from build123d import *

# Parameters (mm, degrees)
F0_R     = 20
F1_DEPTH = 1.5
F2_R     = 17.5
F3_DEPTH = 10
F4_R     = 20
F5_DEPTH = 1.5
F6_R     = 12.5
F7_DEPTH = 5
F8_R     = 4
F9_DEPTH = 20


with BuildPart() as f1:
    # F0 (on Front) → F1 (new body)
    with BuildSketch(Plane.XZ):
        Circle(F0_R)
    extrude(amount=F1_DEPTH)

    # F2 (on face) → F3 (join)
    with BuildSketch(Plane.XZ.offset(1.5)):
        Circle(F2_R)
    extrude(amount=F3_DEPTH)

    # F4 (on face) → F5 (join)
    with BuildSketch(Plane.XZ.offset(11.5)):
        Circle(F4_R)
    extrude(amount=F5_DEPTH)

    # F6 (on face) → F7 (join)
    with BuildSketch(Plane.XZ.offset(13)):
        Circle(F6_R)
    extrude(amount=F7_DEPTH)

    # F8 (on face) → F9 (cut)
    with BuildSketch(Plane.XZ.offset(18)):
        Circle(F8_R)
    extrude(amount=-F9_DEPTH, mode=Mode.SUBTRACT)


solid = f1.part
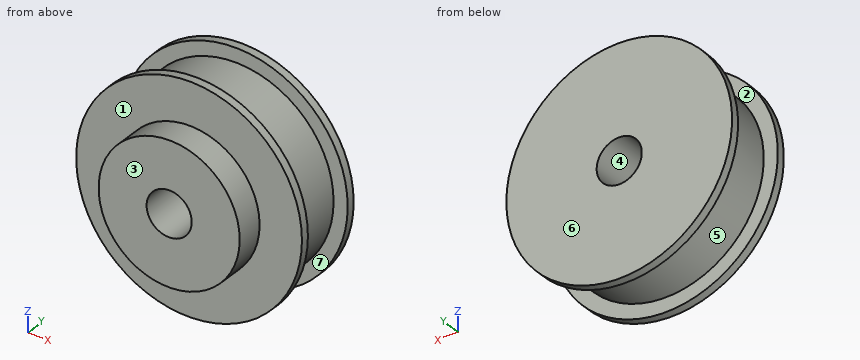
Model file for the job. Use its own axes, mm. Face numbers are marked on the shaded views. A direction names the side the tool comes from. Give positions to 0.01 mm unless a question says otherwise; leave off trailing zeros. Write each loop counter-clockwise with the first axis right and the second up, starting at its lowest first coordinate (ties: lowest second). Pieces come first, ordered by that corner, then holes. Notation, with made-up numbers: (35.5, 2.25) -> (41.5, 2.25) arc R27 ccw to (41.5, 33.25) -> close; hole circle Ø2 at (88.25, 4). An arc over 180 degrees is marked (long way). Write item = value, one per line.
(1) Slice it at C-C, the plane y = -6.5. Give the cut face in (x, z), then the cut area to 3 significant figures.
Determined:
outline = circle Ø35 at (0, 0); hole circle Ø8 at (0, 0)
area = 912 mm2
(2) Slice it at B-B, the plane x = 0. Give the cut face in (y, z).
Determined:
outline = (-18, -12.5) -> (-13, -12.5) -> (-13, -20) -> (-11.5, -20) -> (-11.5, -17.5) -> (-1.5, -17.5) -> (-1.5, -20) -> (0, -20) -> (0, -4) -> (-18, -4) -> close; (-18, 4) -> (0, 4) -> (0, 20) -> (-1.5, 20) -> (-1.5, 17.5) -> (-11.5, 17.5) -> (-11.5, 20) -> (-13, 20) -> (-13, 12.5) -> (-18, 12.5) -> close
(3) Flat gauge pins, fed straight in: P1, Ø4, axis at y = -2, z = -9, coming from the -X side; P2, Ø2, axis at x = -9.5, y = -3.5, coming from the +Z side; P3, Ø1.5, axis at x = 13, z = 5.5, coming from the -Y side; P4, Ø6.5, axis at x = 0, z = 0, coming from the -Y side. Where does each tip first touch, or does it go through?
Determined:
P1 = -18.71
P2 = 15.3
P3 = -13
P4 = through
(4) Probe line 1 along Y through (x, z) = (-6.5, 18); line 2 along Z through (x, y) = (0, -6); line 3 along Y through (x, z) = (-9, -9.5). List the from-to ranges inside material, lowest first.
Determined:
line_1 = -13 to -11.5, -1.5 to 0
line_2 = -17.5 to -4, 4 to 17.5
line_3 = -13 to 0
(5) Tool access for the marked faces 1, 2 and 3: list every direction of +Z, -Z, +X, -X, +Y, -Y with a clear straight run to the whole face (end or side of a thin tool).
Determined:
face_1 = -Y
face_2 = none
face_3 = +Z, -Z, +X, -X, -Y
(6) Slice it at D-D, the plane z = -4.5. Give the cut face in (x, y), then the cut area to 3 significant figures.
Determined:
outline = (-19.49, -13) -> (-11.66, -13) -> (-11.66, -18) -> (11.66, -18) -> (11.66, -13) -> (19.49, -13) -> (19.49, -11.5) -> (16.91, -11.5) -> (16.91, -1.5) -> (19.49, -1.5) -> (19.49, 0) -> (-19.49, 0) -> (-19.49, -1.5) -> (-16.91, -1.5) -> (-16.91, -11.5) -> (-19.49, -11.5) -> close
area = 572 mm2
(7) Slice it at A-A, the plane z = 0. Give the cut face in (x, y).
Determined:
outline = (-20, -13) -> (-12.5, -13) -> (-12.5, -18) -> (-4, -18) -> (-4, 0) -> (-20, 0) -> (-20, -1.5) -> (-17.5, -1.5) -> (-17.5, -11.5) -> (-20, -11.5) -> close; (4, -18) -> (12.5, -18) -> (12.5, -13) -> (20, -13) -> (20, -11.5) -> (17.5, -11.5) -> (17.5, -1.5) -> (20, -1.5) -> (20, 0) -> (4, 0) -> close
(8) Mould opens along Y. For the marked faces 4, 5, 6 and 7 say: released by +Y, released by -Y, zero draft, split by the parting line, or undercut.
Determined:
face_4 = zero draft
face_5 = undercut
face_6 = released by +Y
face_7 = undercut
